Read the model definition and answer for the solid it produces. Units are mm, in the model's axes. A direction names the side the tool comes from. Coordinates: 2 decimals unless noted, no trailing zeros. Write each loop counter-clockwise with the first axis right and the second up, starting at its lowest first coordinate (ties: lowest second). Pieces come first, ordered by that corner, then holes. Notation, with made-up numbers: M 4,26 L 32,26 A23 cw 32,37 Z; hole C 13,9 d11. An arc over 180 degrees is marked long. Write item = value, one per line.
Autodesk Inventor part; units mm, degrees
ref_plane "YZ Plane" through (0, 0, 0) normal (1, 0, 0) x (0, 1, 0)
ref_plane "XZ Plane" through (0, 0, 0) normal (0, 1, 0) x (-1, 0, 0)
ref_plane "XY Plane" through (0, 0, 0) normal (0, 0, 1) x (1, 0, 0)
sketch "Sketch1" plane through (0, 0, 0) normal (1, 0, 0) x (0, 1, 0)
  line L0 (0, 0) -> (-65, 0)
  line L1 (-65, 0) -> (-65, -75)
  line L2 (-65, -75) -> (0, -75)
  line L3 (0, -75) -> (0, 0)
  line L4 (-40.75, -13.75) -> (-48.25, -13.75)
  line L5 (-48.25, -13.75) -> (-48.25, -21.25)
  line L6 (-48.25, -21.25) -> (-40.75, -21.25)
  line L7 (-40.75, -21.25) -> (-40.75, -13.75)
  arc A0 (-40.75, -21.25) -> (-40.75, -13.75) centre (-40.75, -17.5) ccw
  arc A1 (-48.25, -13.75) -> (-48.25, -21.25) centre (-48.25, -17.5) ccw
  line L8 (-40.75, -53.75) -> (-48.25, -53.75)
  line L9 (-48.25, -53.75) -> (-48.25, -61.25)
  line L10 (-48.25, -61.25) -> (-40.75, -61.25)
  line L11 (-40.75, -61.25) -> (-40.75, -53.75)
  arc A2 (-40.75, -61.25) -> (-40.75, -53.75) centre (-40.75, -57.5) ccw
  arc A3 (-48.25, -53.75) -> (-48.25, -61.25) centre (-48.25, -57.5) ccw
  circle A4 centre (-10, -17.5) radius 3.25
  circle A5 centre (-10, -57.5) radius 3.25
  dimension "d1" = 75
  dimension "d4" = 7.5
  dimension "d5" = 7.5
  dimension "d8" = 13.75
  dimension "d10" = 40
  dimension "d15" = 10
  dimension "d16" = 6.5
  dimension "d17" = 6.5
  dimension "d18" = 30.75
  dimension "d19" = 65
  dimension "d20" = 7.5
extrude "Extrusion1" add sketch "Sketch1" along normal blind 6.35
equation "\"d5\" = d4"
equation "\"d8\" = -0.5 * d4 + 0.5 * d1 - 0.5 * d10"
equation "\"d17\" = d16"
properties part number "mounting bracket 1"
Item 1: Which of the six approach directions +Z, -Z, +X, -X, +Y, -Y give full straight-line access (tool end or side, diameter ignored) to faces 4 (the face through (3, -32, 0)), 5 (the face through (3.1, -37, -17.4))?
Worked answers:
face_4 = +Z, +X, -X, +Y, -Y
face_5 = +X, -X
Item 2: Find section B-B (y = -10). Determine the outline of the cut face in (x, z).
Worked answers:
outline = M 0,-75 L 6.35,-75 L 6.35,-60.75 L 0,-60.75 Z; M 0,-54.25 L 6.35,-54.25 L 6.35,-20.75 L 0,-20.75 Z; M 0,-14.25 L 6.35,-14.25 L 6.35,0 L 0,0 Z
Item 3: Consider line 1 along Z through (x, y) = (4.25, -10); line 2 along Z through (x, y) = (2.5, -47.5); line 3 along Y through (x, z) = (3.75, -16). Determine where each line is inside the solid, lowest interval first. Write a range as from..to.
Worked answers:
line_1 = -75..-60.75, -54.25..-20.75, -14.25..0
line_2 = -75..-61.25, -53.75..-21.25, -13.75..0
line_3 = -65..-51.69, -37.31..-12.88, -7.12..0
Item 4: For a pull along Z with two mould halves and no side action, classify faces 1 (the face through (3, -33, -75)), 2 (the face through (3.1, -52, -17.6)), 3 (the face through (0, -33, -37)) as released by +Z, released by -Z, zero draft, split by the parting line, or undercut.
Worked answers:
face_1 = released by -Z
face_2 = undercut
face_3 = zero draft
Item 5: Find section C-C (x = 3.5). Determine the outline of the cut face in (y, z).
Worked answers:
outline = M -65,-75 L 0,-75 L 0,0 L -65,0 Z; hole M -48.25,-61.25 L -40.75,-61.25 A3.75 ccw -40.75,-53.75 L -48.25,-53.75 A3.75 ccw Z; hole M -48.25,-21.25 L -40.75,-21.25 A3.75 ccw -40.75,-13.75 L -48.25,-13.75 A3.75 ccw Z; hole C -10,-57.5 d6.5; hole C -10,-17.5 d6.5
Item 6: Flat-ended cylindrical pins translate along their axes: pin 1 (2 mm diameter, centred on y = -51.5, z = -41, fed in from -X); pin 2 (4 mm diameter, centred on y = -10, z = -57.5, fed in from -X). Find the tip coordinate at first contact, or state that the pin passes through.
Worked answers:
pin_1 = 0
pin_2 = through
Item 7: Find section A-A (z = -17.5). Determine the outline of the cut face in (x, y).
Worked answers:
outline = M 0,-65 L 6.35,-65 L 6.35,-52 L 0,-52 Z; M 0,-37 L 6.35,-37 L 6.35,-13.25 L 0,-13.25 Z; M 0,-6.75 L 6.35,-6.75 L 6.35,0 L 0,0 Z
